Can you work these out from the drawing? Everything is in mm from the part's minimum corner. A direction names the side the tool comes from. Coordinates: 2 decimals unless noted, no trailing zeros. Use one line per item in the form item = value. Start each with the question number.
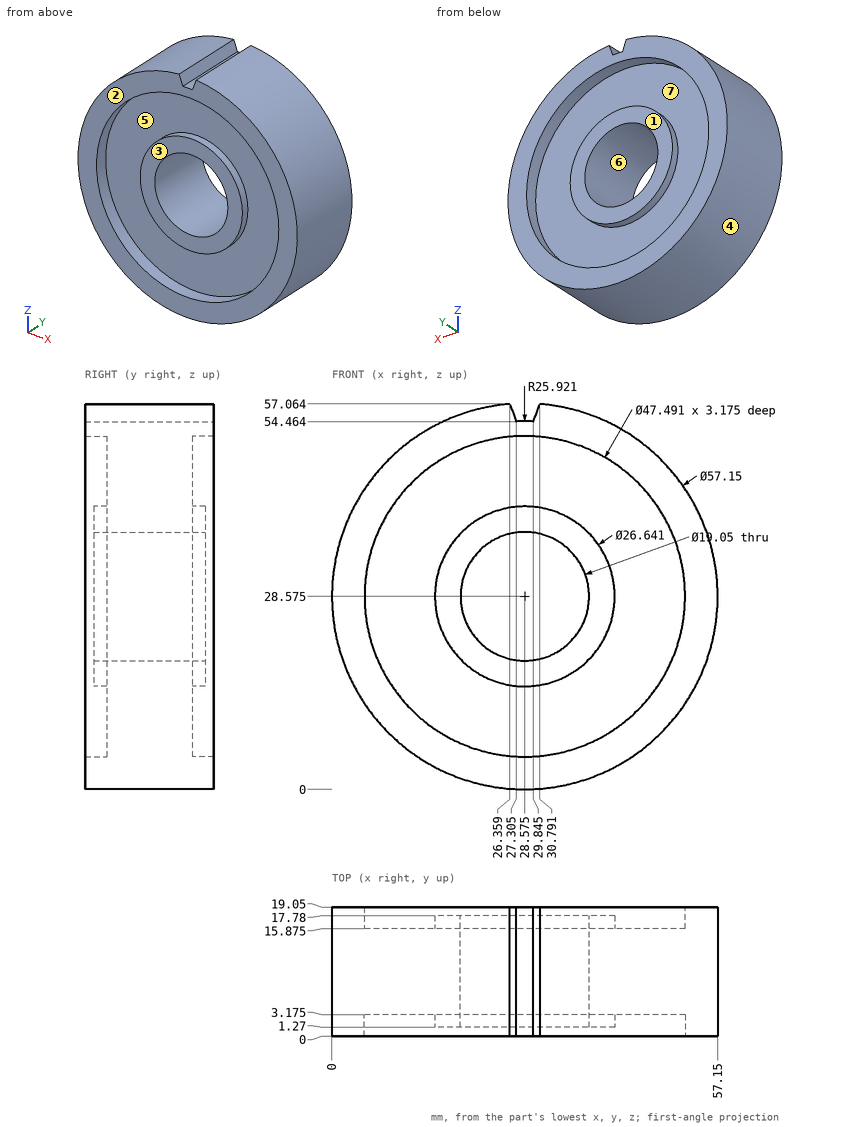
1) For pin 1 (1 mm diameter, centred on x = 28, y = 7.5, fed in from -Z); pin 2 (23.5 mm diameter, centred on x = 24.5, z = 26.5, fed in from +Y); pin 3 (10 mm diameter, centred on x = 8.5, z = 29, fed in from +Y); pin 4 (10 mm diameter, centred on y = 14, z = 7.5, fed in from -X), each with a flat end and sliding along its axis, tell me the tip position at first contact or that it passes through.
2) I need wall thicknesses on probe 1 along Z at (x, y) = (32, 16) (1 decimal); probe 2 along X at (y, z) = (17.5, 26) (1 decimal); probe 3 along Y at (x, z) = (26.5, 40). Which ranges of each line are inside material? Lowest first, please. Write a range as [from, to].
3) If we mould it in two halves opening along Z, with no side actions, what happens to the marked faces 1, 2, 3 and 4? For each: pulls with the +Z half, pulls with the -Z half, needs draft (parallel to the pull), parting line crosses it, or undercut.
4) Which directions (+Z, -Z, +X, -X, +Y, -Y) give clear straight access to the entire face, cutting with the end or side of a thin tool? Please do the marked faces 5, 6 and 7.
From the geometry:
q1.pin_1 = 0
q1.pin_2 = 17.78
q1.pin_3 = 19.05
q1.pin_4 = 4.95
q2.probe_1 = [0.2, 5.1], [15.7, 19.7], [37.5, 41.4], [52.1, 56.9]
q2.probe_2 = [0.1, 5], [15.5, 19.4], [37.7, 41.6], [52.2, 57]
q2.probe_3 = [1.27, 17.78]
q3.face_1 = undercut
q3.face_2 = needs draft
q3.face_3 = undercut
q3.face_4 = parting line crosses it
q4.face_5 = -Y
q4.face_6 = +Y, -Y
q4.face_7 = +Y
